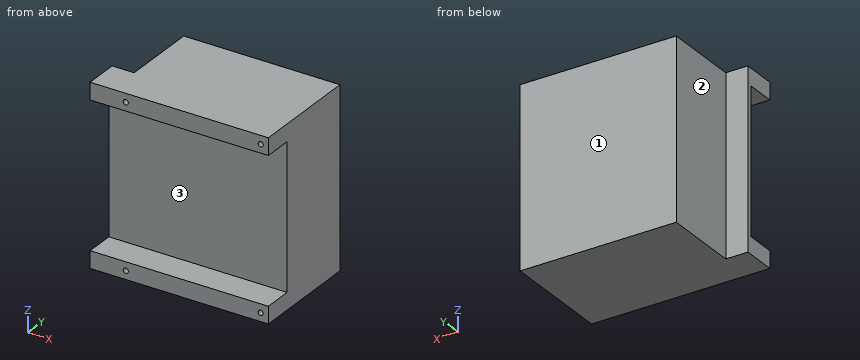
from build123d import *

# Parameters (mm, degrees)
SKETCH1_W           = 92
SKETCH1_H           = 105
BOSS_EXTRUDE1_DEPTH = 45
SKETCH2_W           = 105
SKETCH2_H           = 105
BOSS_EXTRUDE2_DEPTH = 3
SKETCH3_W           = 105
SKETCH3_H           = 10
BOSS_EXTRUDE3_DEPTH = 17
SKETCH4_R           = 1.5
CUT_EXTRUDE1_DEPTH  = 35


with BuildPart() as part:
    # Sketch1 → Boss-Extrude1 (new body)
    with BuildSketch(Plane(origin=(0, 0, 0), x_dir=(1, 0, 0), z_dir=(0, 1, 0))):
        Rectangle(SKETCH1_W, SKETCH1_H)
    extrude(amount=BOSS_EXTRUDE1_DEPTH)

    # Sketch2 → Boss-Extrude2 (add)
    with BuildSketch(Plane.XZ):
        with Locations((-6.5, 0)):
            Rectangle(SKETCH2_W, SKETCH2_H)
    extrude(amount=BOSS_EXTRUDE2_DEPTH)

    # Sketch3 → Boss-Extrude3 (add)
    with BuildSketch(Plane.XZ.offset(3)):
        with Locations((-6.5, 47.5)):
            Rectangle(SKETCH3_W, SKETCH3_H)
    boss_extrude3 = extrude(amount=BOSS_EXTRUDE3_DEPTH)

    # Sketch4 → Cut-Extrude1 (cut)
    with BuildSketch(Plane(origin=(0, -20, 0), x_dir=(-1, 0, 0), z_dir=(0, -1, 0))):
        with Locations(Location((-41.5, -47.5, 0), (0, 0, 90))):
            Circle(SKETCH4_R)
        with Locations(Location((38, -47.5, 0), (0, 0, 90))):
            Circle(SKETCH4_R)
    cut_extrude1 = extrude(amount=-CUT_EXTRUDE1_DEPTH, mode=Mode.SUBTRACT)

    # Mirror1: Boss-Extrude3, Cut-Extrude1 across plane
    add(boss_extrude3.mirror(Plane.XY))
    add(cut_extrude1.mirror(Plane.XY), mode=Mode.SUBTRACT)


solid = part.part
Geometry check sheet. Reference: the model listing, model coordinates, mm. Face numbers are marked on the shaded views. A direction names the side the tool comes from. Round coordinates to 2 decimals unless told otherwise and drop trailing zeros. Loops run counter-clockwise (first coordinate to the right, second up) from the corner with the lowest first, then second, coordinate; pieces in that order, holes last.
Item 1: Cross-section at D-D on x = -25.5. Record the boundary of the cut face in (y, z).
Item 2: Cross-section at A-A on y = 5. Record the boundary of the cut face in (x, z), then the cut area to 3 significant figures.
Item 3: Cross-section at B-B on x = 41.5. Record the boundary of the cut face in (y, z).
Item 4: Gauge pin test, flat ends, axial feed: pin 1 (2.5 mm diameter, centred on x = -38, z = 47.5, fed in from -Y); pin 2 (12 mm diameter, centred on x = -40, z = 26, fed in from -Y); pin 3 (10.5 mm diameter, centred on x = -54.5, z = 20, fed in from +Y). Record the tip position at first contact, or that the pin passes through.
Item 5: Access from +Z, -Z, +X, -X, +Y, -Y to the whole of each face (thin tool, end or side, straight path). Record for the marked faces 1, 2 and 3.
Item 6: Thickness scan on line 1 (X direction, y = -7, z = 47.5); line 2 (X direction, y = 5.5, z = 47.5); line 3 (Z direction, x = 41, y = 0). Record the ranges inside material, lowest first.
Item 7: Cross-section at C-C on z = 47.5. Record the boundary of the cut face in (x, y), then the cut area to 3 significant figures.
Answer sheet:
1. outline: (-20, -52.5) - (45, -52.5) - (45, 52.5) - (-20, 52.5) - (-20, 42.5) - (-3, 42.5) - (-3, -42.5) - (-20, -42.5) - close
2. outline: (-46, -52.5) - (46, -52.5) - (46, 52.5) - (-46, 52.5) - close; hole circle Ø3 at (-38, -47.5); hole circle Ø3 at (-38, 47.5); hole circle Ø3 at (41.5, -47.5); hole circle Ø3 at (41.5, 47.5)
2. area: 9,630 mm2
3. outline: (-20, -52.5) - (45, -52.5) - (45, 52.5) - (-20, 52.5) - (-20, 49) - (15, 49) - (15, 46) - (-20, 46) - (-20, 42.5) - (-3, 42.5) - (-3, -42.5) - (-20, -42.5) - (-20, -46) - (15, -46) - (15, -49) - (-20, -49) - close
4. pin 1: stops at y = 15
4. pin 2: stops at y = -3
4. pin 3: stops at y = 0
5. face 1: +Z, -Z, +X, -X, +Y
5. face 2: +Z, -Z, -X, +Y
5. face 3: +X, -X, -Y
6. line 1: x = -59 to -39.5, -36.5 to 40, 43 to 46
6. line 2: x = -46 to -39.5, -36.5 to 40, 43 to 46
6. line 3: z = -52.5 to -48.91, -46.09 to 46.09, 48.91 to 52.5
7. outline: (-59, -20) - (-39.5, -20) - (-39.5, 15) - (-36.5, 15) - (-36.5, -20) - (40, -20) - (40, 15) - (43, 15) - (43, -20) - (46, -20) - (46, 45) - (-46, 45) - (-46, 0) - (-59, 0) - close
7. area: 6,030 mm2
